from build123d import *

# Parameters (mm, degrees)
SKETCH016_R     = 2.4
PAD017_DEPTH    = 20
SKETCH020_W     = 2.5
SKETCH020_H     = 16.93
PAD021_DEPTH    = 18.3
POCKET002_DEPTH = 20
POCKET004_DEPTH = 20.001
PAD029_DEPTH    = 16.4
POCKET013_DEPTH = 18.95102
SKETCH036_R     = 2.1
POCKET014_DEPTH = 13.861
SKETCH037_R     = 2.1
POCKET015_DEPTH = 5.501
SKETCH045_R     = 0.9
POCKET016_DEPTH = 18.861


with BuildPart() as corner_front_left:
    # Sketch016 → Pad017 (new body)
    with BuildSketch(Plane.XY):
        with BuildLine():
            ThreePointArc((-121.92, -35.56), (-116.758725, -45.780451), (-105.46998, -47.693728))
            Line((-105.46998, -46.223728), (-105.46998, -47.693728))
            Line((-111.96998, -46.223728), (-105.46998, -46.223728))
            Line((-111.96998, -43.123728), (-111.96998, -46.223728))
            Line((-105.46998, -43.123728), (-111.96998, -43.123728))
            Line((-105.46998, -31.693728), (-105.46998, -43.123728))
            Line((-105.46998, -31.693728), (-105.46998, -26.193728))
            ThreePointArc((-105.46998, -26.193728), (-105.669987, -25.66457), (-106.17, -25.4))
            Line((-106.17, -25.4), (-121.92, -25.4))
            Line((-121.92, -25.4), (-121.92, -35.56))
        make_face()
        with Locations((-109.22, -35.56)):
            Circle(SKETCH016_R, mode=Mode.SUBTRACT)
    extrude(amount=PAD017_DEPTH)

    # Sketch020 (on Face13 of Pad017) → Pad021 (join)
    with BuildSketch(Plane.XY.offset(20)):
        with Locations((-104.21998, -34.658728)):
            Rectangle(SKETCH020_W, SKETCH020_H)
    extrude(amount=-PAD021_DEPTH)

    # Sketch028 (on Face15 of Pad021) → Pocket002 (cut)
    with BuildSketch(Plane.XY.offset(20)):
        Polygon((-106.47, -37.147713), (-106.47, -33.972287), (-109.22, -32.384574), (-111.97, -33.972287), (-111.97, -37.147713), (-109.22, -38.735426), align=None)
    extrude(amount=-POCKET002_DEPTH, mode=Mode.SUBTRACT)

    # Sketch031 (on Face19 of Pocket002) → Pocket004 (cut, through all)
    with BuildSketch(Plane.XY.offset(20)):
        Polygon((-121.92, -25.4), (-109.17, -25.4), (-106.17, -29.4), (-121.92, -29.4), align=None)
    extrude(amount=-POCKET004_DEPTH, mode=Mode.SUBTRACT)

    # Sketch032 (on Face21 of Pocket004) → Pad029 (join)
    with BuildSketch(Plane.XY.offset(20)):
        with BuildLine():
            Line((-119.92, -29.4), (-119.92, -28.9))
            ThreePointArc((-119.827265, -28.47944), (-119.896541, -28.684669), (-119.92, -28.9))
            ThreePointArc((-111.555319, -27.001504), (-116.075974, -25.587421), (-119.827265, -28.47944))
            ThreePointArc((-111.555319, -27.001504), (-110.411621, -26.986272), (-110.452117, -25.843189))
            ThreePointArc((-110.452117, -25.843189), (-116.463348, -23.966517), (-121.764907, -27.365086))
            ThreePointArc((-121.764907, -27.365086), (-121.880444, -27.621528), (-121.92, -27.9))
            Line((-121.92, -27.9), (-121.92, -29.4))
            Line((-121.92, -29.4), (-121.92, -30.4))
            Line((-121.92, -30.4), (-119.92, -30.4))
            Line((-119.92, -30.4), (-119.92, -29.4))
        make_face()
    extrude(amount=-PAD029_DEPTH)

    # Sketch034 (on Plane of DatumPlane001) → Pocket013 (cut, through all)
    with BuildSketch(Plane(origin=(-121.92, 0, 0), x_dir=(0, -1, 0), z_dir=(-1, 0, 0))):
        with BuildLine():
            Line((26.9, 20), (26.9, 21))
            Line((26.9, 21), (22.9, 21))
            Line((22.9, 21), (22.9, 17))
            Line((22.9, 17), (23.9, 17))
            ThreePointArc((26.9, 20), (24.77868, 19.12132), (23.9, 17))
        make_face()
    extrude(amount=-POCKET013_DEPTH, mode=Mode.SUBTRACT)

    # Sketch036 (on Face8 of Pocket013) → Pocket014 (cut, through all)
    with BuildSketch(Plane(origin=(0, -34.4, 0), x_dir=(-1, 0, 0), z_dir=(0, 1, 0))):
        with Locations((114.3, 8)):
            Circle(SKETCH036_R)
    extrude(amount=-POCKET014_DEPTH, mode=Mode.SUBTRACT)

    # Sketch037 (on Face8 of Pocket014) → Pocket015 (cut, through all)
    with BuildSketch(Plane(origin=(0, -29.4, 0), x_dir=(-1, 0, 0), z_dir=(0, 1, 0))):
        with Locations((114.3, 8)):
            Circle(SKETCH037_R)
    extrude(amount=POCKET015_DEPTH, mode=Mode.SUBTRACT)

    # Sketch045 (on Face8 of Pocket015) → Pocket016 (cut, through all)
    with BuildSketch(Plane(origin=(0, -29.4, 0), x_dir=(-1, 0, 0), z_dir=(0, 1, 0))):
        with Locations((114.3, 8)):
            Circle(SKETCH045_R)
    extrude(amount=-POCKET016_DEPTH, mode=Mode.SUBTRACT)


with BuildPart() as corner_front_left_1:
    # Body012 placement: moved
    add(corner_front_left.part.moved(Location((0, 19, 0))))


with BuildPart() as corner_front_right_mirrored:
    # mirror: instance of Corner_front_left
    add(corner_front_left_1.part.mirror(Plane(origin=(1e-06, -17.077076, 10), x_dir=(0, -1, 0), z_dir=(1, 0, 0))))


solid = corner_front_right_mirrored.part
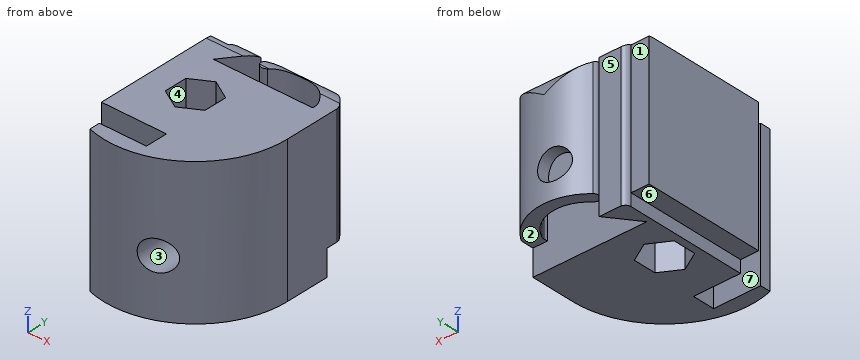
Check sheet for the modelled part. Datum: model origin and axes. Units: mm. Face numbers are marked on the shaded views. A direction names the side the tool comes from. Give positions to 0.01 mm unless a question says otherwise; leave off trailing zeros. Write each loop counter-clockwise with the first axis right and the second up, starting at its lowest first coordinate (ties: lowest second). Pieces come first, ordered by that corner, then holes. Notation, with made-up numbers: (72, 83.25) -> (80, 83.25) arc R35 cw to (80, 121.25) -> close; hole circle Ø11 at (85.5, 55.5). An arc over 180 degrees is marked (long way). One line per item, written item: value. Start each with the question number.
Item 1: Draft check along Z on the marked faces 1, 2 and 3. Enter one of: +Z half, -Z half, draft (parallel to the pull), parting line (faces both ways), or undercut.
Item 2: Section check B-B on y = -11.5. Record the cut outline in (x, z).
Item 3: Tool access check on the marked faces 4, 5, 6 and 7. Record the directions out of +Z, -Z, +X, -X, +Y, -Y that give a thin tool (end or side, any length) a straight path to the whole face; none if there is none.
Item 4: Section check A-A on z = 2. Record the cut outline in (x, y), then the cut area to 3 significant figures.
Item 5: Gauge pin test, flat ends, axial feed: pin 1 (2.5 mm diameter, centred on x = 109.5, z = 14, fed in from -Y); pin 2 (4 mm diameter, centred on x = 118, z = 4, fed in from -Y); pin 3 (3.5 mm diameter, centred on x = 113.5, z = 8, fed in from -Y); pin 4 (12 mm diameter, centred on y = -24.5, z = 15, fed in from +X). Record the tip position at first contact, or that the pin passes through.
Item 6: Material ranges on probe 1 along Z at (x, y) = (114.25, -16.75); probe 2 along Y at (x, z) = (110.75, 7); probe 3 along Y at (x, z) = (108.25, 14), recorded low to high. Write a range as from..to.
Item 7: Section check C-C on z = 8.5. State how many separate pieces and enclosed holes the cut face has, then the cut area to 3 significant figures.
Item 8: Section check D-D on x = 120.75. Record the cut outline in (y, z).
Results list:
1. face 1: draft
1. face 2: -Z half
1. face 3: undercut
2. outline: (102.97, 1.7) -> (105.47, 1.7) -> (105.47, 0) -> (121.92, 0) -> (121.92, 20) -> (102.97, 20) -> close; hole circle Ø1.8 at (114.3, 8)
3. face 4: +Z, -Z
3. face 5: +Z, -Z, -X, +Y
3. face 6: -Z, -X, +Y, -Y
3. face 7: +Z, -Z, -X
4. outline: (102.97, -24.12) -> (111.97, -24.12) -> (111.97, -27.22) -> (105.47, -27.22) -> (105.47, -28.69) arc R12.7 ccw to (121.92, -16.56) -> (121.92, -10.4) -> (106.17, -10.4) -> (109.17, -6.4) -> (106.17, -6.4) arc R0.8 ccw to (105.47, -7.19) -> (102.97, -7.19) -> close; hole (106.47, -18.15) -> (109.22, -19.74) -> (111.97, -18.15) -> (111.97, -14.97) -> (109.22, -13.38) -> (106.47, -14.97) -> close
4. area: 280 mm²
5. pin 1: y = -29.26
5. pin 2: y = -27.3
5. pin 3: y = -29.01
5. pin 4: x = 121.77
6. probe 1: 0..5.9, 10.1..20
6. probe 2: -29.17..-27.22, -24.12..-18.85, -14.27..-10.4, -8.2..-6.59
6. probe 3: -29.22..-27.22, -24.12..-19.18, -13.94..-10.4, -7.63..-6.4
7. separate pieces: 3
7. enclosed holes: 1
7. area: 238 mm²
8. outline: (-21.88, 0) -> (-10.4, 0) -> (-10.4, 3.6) -> (-7.09, 3.6) -> (-7.09, 19.89) arc R3 ccw to (-7.9, 20) -> (-21.88, 20) -> close
